from build123d import *

# Parameters (mm, degrees)
F0_W     = 50.8
F0_H     = 38.1
F1_DEPTH = 31.75
F3_DEPTH = 50.801
F4_W     = 25.4
F4_H     = 11.23293
F5_DEPTH = 31.751


with BuildPart() as f1:
    # F0 (on Front) → F1 (new body)
    with BuildSketch(Plane.XZ):
        with Locations((-0.257215, 19.05)):
            Rectangle(F0_W, F0_H)
    extrude(amount=F1_DEPTH)

    # F2 (on face) → F3 (cut, through all)
    with BuildSketch(Plane.YZ.offset(25.142785)):
        with BuildLine():
            ThreePointArc((-31.75, 12.7), (-13.789488, 20.139488), (-6.35, 38.1))
            Line((-6.35, 38.1), (-31.75, 38.1))
            Line((-31.75, 38.1), (-31.75, 12.7))
        make_face()
    extrude(amount=-F3_DEPTH, mode=Mode.SUBTRACT)

    # F4 (on face) → F5 (cut, through all)
    with BuildSketch(Plane.XZ.offset(31.75)):
        with Locations((-0.257215, 32.516378)):
            Rectangle(F4_W, F4_H)
    extrude(amount=-F5_DEPTH, mode=Mode.SUBTRACT)


solid = f1.part
Read the model definition and answer for the solid it produces. Units are mm, in the model's axes. A direction names the side the tool comes from. Round coordinates to 2 decimals unless told otherwise and drop trailing zeros. Write each loop counter-clockwise with the first axis right and the second up, starting at its lowest first coordinate (ties: lowest second). Pieces come first, ordered by that corner, then holes.
1. The part is cut by section B-B, the plane y = -2.5. Determine the outline of the cut face in (x, z), then the cut area to 3 significant figures.
2. The part is cut by section A-A, the plane z = 33.5. Determine the outline of the cut face in (x, y).
3. Determine the mould class of faces 1 (the face through (-1, -31.75, 6)), 2 (the face through (12.443, -4, 32)), 3 (the face through (25.143, -12, 15)) for opening direction X: pulls with the +X half, pulls with the -X half, needs draft (parallel to the pull), parting line crosses it, or undercut.
4. Which of the six approach directions +Z, -Z, +X, -X, +Y, -Y give full straight-line access (tool end or side, diameter ignored) to faces 4 (the face through (-12.957, -4, 32)), 5 (the face through (19, -3, 38.1))?
5. The part is cut by section D-D, the plane x = 17.5. Determine the outline of the cut face in (y, z).
6. Straight lines are drawn through the part: L1, parallel to Z at x = -1.5, y = -1; L2, parallel to Y at x = 7.5, z = 18.5; L3, parallel to Z at x = 5.5, y = -17. For each, find the intervals that lie inside material, in ascending order.
7. Given pin 1 Ø10 at (x, y) = (4, -4) entering from +Z; pin 2 Ø1.5 at (x, z) = (18, 19.5) entering from -Y, each flat-ended and moving along its own axis, determine where each tip first touches the part or whether it passes through.
8. The part is cut by section C-C, the plane x = -0.5. Determine the outline of the cut face in (y, z).
Values:
1. outline: (-25.66, 0) - (25.14, 0) - (25.14, 38.1) - (12.44, 38.1) - (12.44, 26.9) - (-12.96, 26.9) - (-12.96, 38.1) - (-25.66, 38.1) - close
1. area: 1,650 mm2
2. outline: (-25.66, -6.77) - (-12.96, -6.77) - (-12.96, 0) - (-25.66, 0) - close; (12.44, -6.77) - (25.14, -6.77) - (25.14, 0) - (12.44, 0) - close
3. face 1: needs draft
3. face 2: undercut
3. face 3: pulls with the +X half
4. face 4: +Z, +Y, -Y
4. face 5: +Z, +X, -X, +Y, -Y
5. outline: (-31.75, 0) - (0, 0) - (0, 38.1) - (-6.35, 38.1) arc R25.4 cw to (-31.75, 12.7) - close
6. L1: z = 0 to 26.9
6. L2: y = -15.59 to 0
6. L3: z = 0 to 17.42
7. pin 1: stops at z = 26.9
7. pin 2: stops at y = -15.3
8. outline: (-31.75, 0) - (0, 0) - (0, 26.9) - (-8.95, 26.9) arc R25.4 cw to (-31.75, 12.7) - close
